Verification items for this drawing (mm, ordinates from the low corner). A direction names the side the tool comes from. Round coordinates to 2 decimals unless told otherwise and drop trailing zeros. Order: outer loops, then holes, each group sorted by start corner. A loop starts at its lowest first (then second) coordinate and runs counter-clockwise, first axis right, second up. Notation, with made-up numbers: M 53.25,51 L 111.25,51 A25 ccw 111.25,74 Z; hole C -14.75,-10 d10. An arc over 180 degrees is marked long. One line per item, written item: value. Start each with the question number.
(1) Cross-section at C-C, the plane y = 17. Enter the section's corners in (x, z).
(2) Depth check by flat-ended pin: pin 1 Ø2 at (x, y) = (150.5, 18) entering from +Z. Enter the tip coordinate at first touch or a pass-through.
(3) Cross-section at B-B, the plane x = 211.5. Enter the section's corners in (y, z) (1 decimal), and give its area (3 significant figures).
(4) Access from +Z, -Z, +X, -X, +Y, -Y to the whole of each face (thin tool, end or side, straight path). Record for the marked faces 5, 6 and 7.
(5) Thickness scan on L1, parallel to X at y = 6.5, z = 103; L2, parallel to X at y = 69.5, z = 62; L3, parallel to Y at x = 89, z = 133. Record the ranges inside material, lowest first.
(6) Cross-section at A-A, the plane z = 96. Enter the section's corners in (x, y).
(7) Cross-section at D-D, the plane x = 140.5. Enter the section's corners in (y, z), and give its area (3 significant figures).
(8) Release check for a two-part mould opening along X. For the marked faces 1, 2, 3 and 4 record: released by +X, released by -X, zero draft, split by the parting line, or undercut.
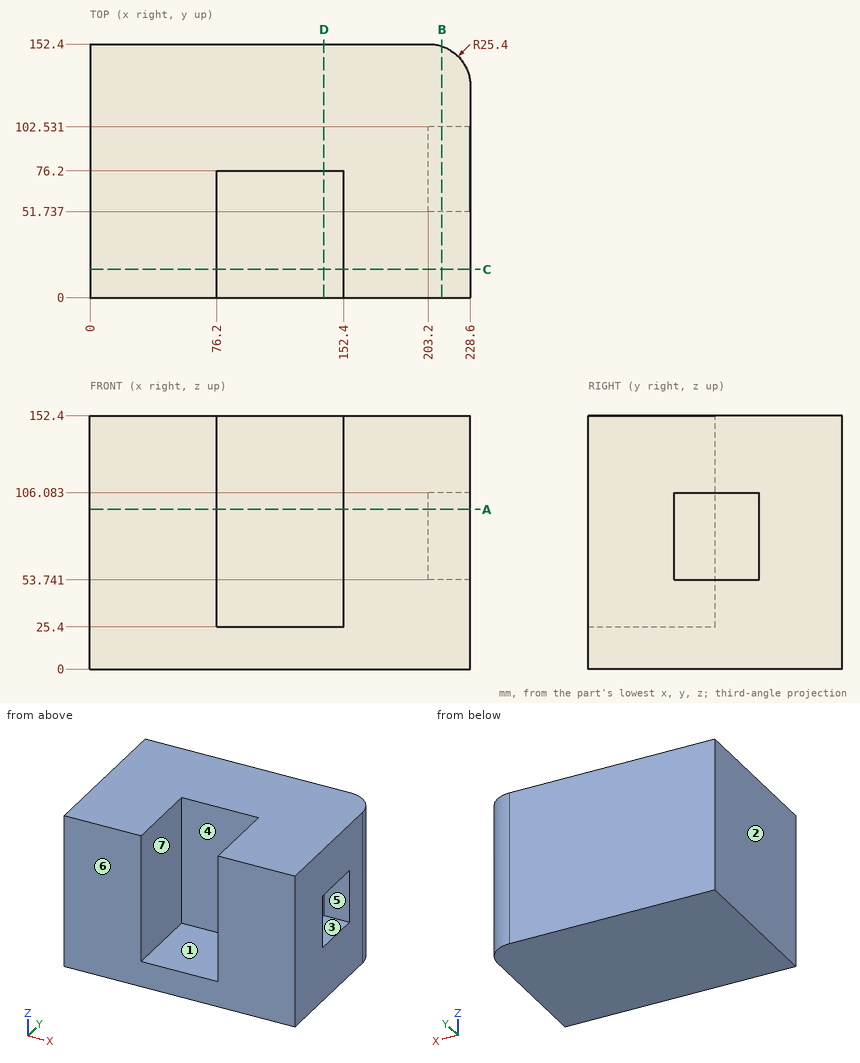
Values found:
1. outline: M 0,0 L 228.6,0 L 228.6,152.4 L 152.4,152.4 L 152.4,25.4 L 76.2,25.4 L 76.2,152.4 L 0,152.4 Z
2. pin 1: z = 25.4
3. outline: M 0,0 L 151,0 L 151,152.4 L 0,152.4 Z; hole M 51.7,53.7 L 102.5,53.7 L 102.5,106.1 L 51.7,106.1 Z
3. area: 20,400 mm^2
4. face 5: +X
4. face 6: +Z, -Z, +X, -X, -Y
4. face 7: +Z, -Y
5. L1: 0 to 76.2, 152.4 to 228.6
5. L2: 0 to 76.2, 152.4 to 203.2
5. L3: 76.2 to 152.4
6. outline: M 0,0 L 76.2,0 L 76.2,76.2 L 152.4,76.2 L 152.4,0 L 228.6,0 L 228.6,51.74 L 203.2,51.74 L 203.2,102.53 L 228.6,102.53 L 228.6,127 A25.4 ccw 203.2,152.4 L 0,152.4 Z
7. outline: M 0,0 L 152.4,0 L 152.4,152.4 L 76.2,152.4 L 76.2,25.4 L 0,25.4 Z
7. area: 13,500 mm^2
8. face 1: undercut
8. face 2: released by -X
8. face 3: zero draft
8. face 4: undercut
